from build123d import *

# Parameters (mm, degrees)
EXTRUDE1_DEPTH  = 170
LPATTERN1_COUNT = 5
LPATTERN1_PITCH = 60


with BuildPart() as part:
    # 15mm → Extrude1 (new, symmetric)
    with BuildSketch(Plane.XY):
        with BuildLine():
            Line((4.949972, 7.600006), (6.192321846, 7.599996))
            ThreePointArc((6.192321846, 7.599996), (6.706266371, 6.946742527), (7.49999, 6.7))
            Line((7.49999, 6.7), (7.49999, 1.000024142))
            Line((7.49999, 1.000024142), (6.499965858, 0))
            Line((6.499965858, 0), (-6.499965858, 0))
            Line((-6.499965858, 0), (-7.49999, 1.000024142))
            Line((-7.49999, 1.000024142), (-7.49999, 6.7))
            ThreePointArc((-7.49999, 6.7), (-6.70626637, 6.946742527), (-6.192321846, 7.599996))
            Line((-6.192321846, 7.599996), (-4.949982, 7.599996))
            Line((-4.949982, 7.599996), (-4.949972, 8.600006))
            Line((-4.949972, 8.600006), (-6.192326435, 8.600016))
            ThreePointArc((-6.192326435, 8.600016), (-6.706271662, 9.253261115), (-7.49999, 9.5))
            Line((-7.49999, 9.5), (-7.49999, 11.099974))
            ThreePointArc((-7.49999, 11.099974), (-6.510037425, 11.510033031), (-6.099989, 12.49999))
            Line((-6.099989, 12.49999), (6.099989, 12.49999))
            ThreePointArc((6.099989, 12.49999), (6.510037425, 11.510033031), (7.49999, 11.099974))
            Line((7.49999, 11.099974), (7.49999, 9.5))
            ThreePointArc((7.49999, 9.5), (6.706271662, 9.253261115), (6.192326435, 8.600016))
            Line((6.192326435, 8.600016), (4.949982, 8.600016))
            Line((4.949982, 8.600016), (4.949972, 7.600006))
        make_face()
    extrude(amount=EXTRUDE1_DEPTH, both=True)

    # Sketch1 → Cut-Revolve1 (revolve, cut)
    with BuildSketch(Plane(origin=(0, 0, 0), x_dir=(0, 0, -1), z_dir=(1, 0, 0))):
        Polygon((-150, 12.49999), (-146.25, 12.49999), (-146.25, 7.19999), (-147.75, 7.19999), (-147.75, 0), (-150, 0), align=None)
    revolve(axis=Axis((0, 0, 150), (0, 1, 0)), mode=Mode.SUBTRACT)

    # Sketch2 → Cut-Revolve2 (revolve, cut)
    with BuildSketch(Plane(origin=(0, 0, 0), x_dir=(0, 0, -1), z_dir=(1, 0, 0))):
        Polygon((150, 0), (152.25, 0), (152.25, 7.19999), (153.75, 7.19999), (153.75, 12.49999), (150, 12.49999), align=None)
    cut_revolve2 = revolve(axis=Axis((0, 12.49999, -150), (0, -1, 0)), mode=Mode.SUBTRACT)

    # LPattern1: Cut-Revolve2 ×5
    with Locations(*[(0, 0, i * LPATTERN1_PITCH) for i in range(1, LPATTERN1_COUNT)]):
        add(cut_revolve2, mode=Mode.SUBTRACT)


solid = part.part
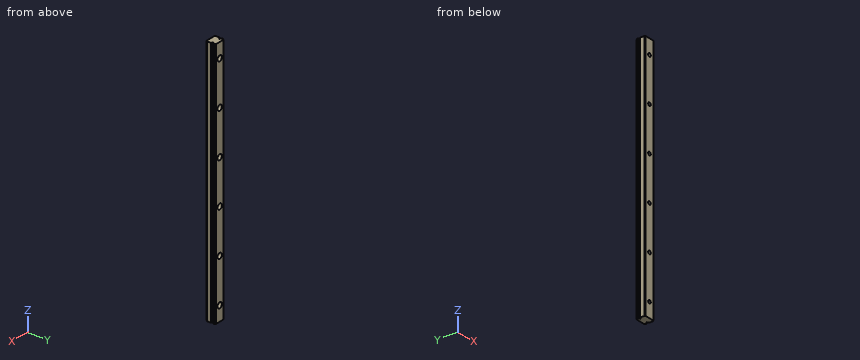
Can you work these out from the model? Positions are in its coordinate system, mm. Coordinates: 2 decimals unless noted, no trailing zeros. Loops run counter-clockwise (first coordinate to the right, second up) from the corner with the lowest first, then second, coordinate; pieces in that order, holes last. Notation, with made-up numbers: M 49,0 L 74,0 A19 cw 74,23 Z; hole C -33,-28 d4. An arc over 180 degrees is marked long. Return JSON: item names as keys, results as strings. Group by question number.
Item 1: If I drill on L1, parallel to Y at x = 5.25, z = 118.5; L2, parallel to X at y = 2, z = -30; L3, parallel to X at y = 8.95, z = 150, over which ranges is the centre line in solid material (lowest first)? Write a range as from..to.
Item 2: Imagine slicing it at A-A (x = 0). Give the number of separate pieces and of enclosed holes in the cut face, and give its area (3 significant figures).
Item 3: I'm going to push a flat-ended pin straight in: pin 1 Ø4 at (x, z) = (0, 151.5) entering from +Y. Where does the tip first touch, or does it pass through?
Item 4: Imagine slicing it at B-B (z = -97.5). Please give me the cut outline in (x, y).
Verdict:
{
 "1": {"L1": "y = 0..7.6, 8.6..12.5", "L2": "x = -7.5..-2.25, 2.25..7.5", "L3": "x = -6.39..-3.75, 3.75..6.39"},
 "2": {"separate pieces": "7", "enclosed holes": "0", "area": "3,820 mm^2"},
 "3": {"pin 1": "stops at y = 7.2"},
 "4": {"outline": "M -7.5,1 L -6.5,0 L 6.5,0 L 7.5,1 L 7.5,6.7 A1.4 cw 6.19,7.6 L 4.95,7.6 L 4.95,8.6 L 6.19,8.6 A1.4 cw 7.5,9.5 L 7.5,11.1 A1.4 cw 6.1,12.5 L -6.1,12.5 A1.4 cw -7.5,11.1 L -7.5,9.5 A1.4 cw -6.19,8.6 L -4.95,8.6 L -4.95,7.6 L -6.19,7.6 A1.4 cw -7.5,6.7 Z"}
}
